```python
from build123d import *

# Parameters (mm, degrees)
F0_W     = 83.5164114833
F0_H     = 55.4486140609
F0_W_2   = 76.1848241091
F0_H_2   = 46.8833819032
F1_DEPTH = 50.8
F2_R     = 9.0216673632
F3_DEPTH = 113.284
F4_W     = 41.1206781864
F4_H     = 16.6921509981
F5_DEPTH = 1117.6


with BuildPart() as f1:
    # F0 (on Front) → F1 (new body)
    with BuildSketch(Plane.XZ):
        with Locations((1.4344416559, 0.6762035191)):
            Rectangle(F0_W, F0_H)
        with Locations((1.2750588357, 1.3524033129)):
            Rectangle(F0_W_2, F0_H_2, mode=Mode.SUBTRACT)
    extrude(amount=F1_DEPTH)

    # F2 (on face) → F3 (cut)
    with BuildSketch(Plane.YZ.offset(43.1926473975)):
        with Locations((-27.8919320554, 0)):
            Circle(F2_R)
    extrude(amount=-F3_DEPTH, mode=Mode.SUBTRACT)

    # F4 (on face) → F5 (cut)
    with BuildSketch(Plane(origin=(0, 0, -27.0481035113), x_dir=(1, 0, 0), z_dir=(0, 0, -1))):
        with Locations((2.2313538939, 42.4539245009)):
            Rectangle(F4_W, F4_H)
    extrude(amount=-F5_DEPTH, mode=Mode.SUBTRACT)


solid = f1.part
```
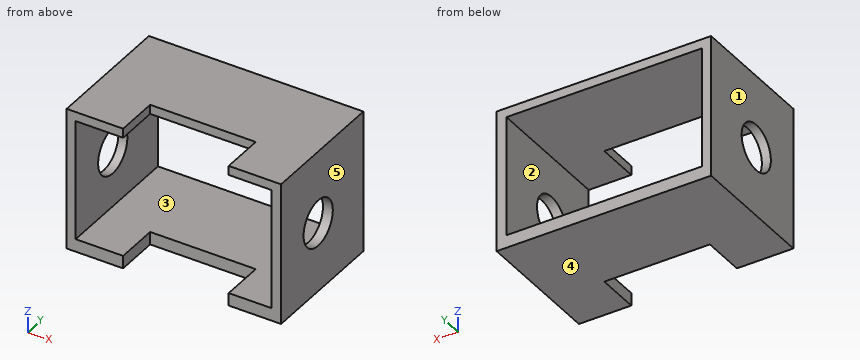
Input: part model. Units: mm. Frame: model coordinates. Face numbers are marked on the shaded views. A direction names the side the tool comes from. Give positions to 0.01 mm unless a question says otherwise; leave off trailing zeros. Order: outer loops, then holes, each group sorted by start corner. A loop starts at its lowest first (then second) coordinate and runs counter-clockwise, first axis right, second up. Notation, with made-up numbers: (38, 0.25) -> (60, 0.25) arc R32 cw to (60, 29.25) -> close; hole circle Ø9 at (-34.75, -4). An arc over 180 degrees is marked (long way). Write each question's results on one line, items separated by ' | '. Start each with the question number.
Item 1: Cut plane A-A on x = -7. Return the cut outline in (y, z).
Item 2: Contact query for flat-ended pins moving along their axis: P1, Ø16, axis at y = -27.89, z = 0, coming from the +X side; P2, Ø1.1, axis at x = -1, z = 26, coming from the -Y side. Output: stop coordinate, or through.
Item 3: Mould query, pull axis X, two halves, no side actions, for the marked faces 3, 4 and 5. Classes: pulls with the +X half, pulls with the -X half, needs draft (parallel to the pull), parting line crosses it, or undercut.
Item 4: Cut plane B-B on z = -19.5. Return the cut outline in (x, y).
Item 5: Cut plane D-D on z = 0. Return the cut outline in (x, y), then the cut area to 3 significant figures.
Item 6: Line query: line 1 (X direction, y = -25, z = 18.5); line 2 (Z direction, x = -33, y = -30.5); line 3 (X direction, y = -38.5, z = -22.5). Output: solid intervals per line, ascending.
Item 7: Set-up query: the marked faces 1 and 2. Return all of +Z, -Z, +X, -X, +Y, -Y with unobstructed straight access to the full face (end or side cutting, diameter ignored); none if empty.
Item 8: Cut plane C-C on y = -40. Return the cut outline in (x, z).
Established:
1) outline: (-34.11, -27.05) -> (0, -27.05) -> (0, -22.09) -> (-34.11, -22.09) -> close; (-34.11, 24.79) -> (0, 24.79) -> (0, 28.4) -> (-34.11, 28.4) -> close
2) P1: through | P2: y = -34.11
3) face 3: undercut | face 4: needs draft | face 5: pulls with the +X half
4) outline: (-40.32, -50.8) -> (-36.82, -50.8) -> (-36.82, 0) -> (-40.32, 0) -> close; (39.37, -50.8) -> (43.19, -50.8) -> (43.19, 0) -> (39.37, 0) -> close
5) outline: (-40.32, -50.8) -> (-36.82, -50.8) -> (-36.82, -36.91) -> (-40.32, -36.91) -> close; (-40.32, -18.87) -> (-36.82, -18.87) -> (-36.82, 0) -> (-40.32, 0) -> close; (39.37, -50.8) -> (43.19, -50.8) -> (43.19, -36.91) -> (39.37, -36.91) -> close; (39.37, -18.87) -> (43.19, -18.87) -> (43.19, 0) -> (39.37, 0) -> close | area: 240 mm^2
6) line 1: -40.32 to -36.82, 39.37 to 43.19 | line 2: -27.05 to -22.09, 24.79 to 28.4 | line 3: -40.32 to -18.33, 22.79 to 43.19
7) face 1: +Z, -Z, -X, +Y, -Y | face 2: +Y, -Y
8) outline: (-40.32, -27.05) -> (-18.33, -27.05) -> (-18.33, -22.09) -> (-36.82, -22.09) -> (-36.82, 24.79) -> (-18.33, 24.79) -> (-18.33, 28.4) -> (-40.32, 28.4) -> close; (22.79, -27.05) -> (43.19, -27.05) -> (43.19, 28.4) -> (22.79, 28.4) -> (22.79, 24.79) -> (39.37, 24.79) -> (39.37, -22.09) -> (22.79, -22.09) -> close
